Geometry check sheet. Reference: drawing and pictorial views, mm from the part's lowest x, y, z. A direction names the side the tool comes from. Round coordinates to 2 decimals unless told otherwise and drop trailing zeros. Order: outer loops, then holes, each group sorted by start corner. A loop starts at its lowest first (then second) coordinate and runs counter-clockwise, first axis right, second up. Notation, with made-up numbers: (-29.5, 54.5) -> (-4.5, 54.5) arc R25 ccw to (-4.5, 76.5) -> close; hole circle Ø7 at (44, 77.25). An arc over 180 degrees is marked (long way). Return JSON: item names as keys, results as strings. Group by question number.
1) Scan lines: L1, parallel to Z at x = 15, y = 1.5; L2, parallel to X at y = 0.8, z = 13; L3, parallel to X at y = 29.45, z = 20. Record each from-to range of solid material in increasing order.
2) Section check D-D on z = 17.5. Enter the section's corners in (x, y).
3) Depth check by flat-ended pin: pin 1 (2.5 mm diameter, centred on x = 25, z = 20, fed in from +Y). Enter the tip coordinate at first touch or a pass-through.
4) Section check A-A on y = 7.25. Enter the section's corners in (x, z).
5) Tool access check on the marked faces 1 and 2. Record the directions out of +Z, -Z, +X, -X, +Y, -Y that give a thin tool (end or side, any length) a straight path to the whole face; none if there is none.
6) Section check B-B on x = 5. Enter the section's corners in (y, z), plus the area to 3 significant figures.
7) Draft check along X on the marked faces 3, 4 and 5. Enter one of: pulls with the +X half, pulls with the -X half, needs draft (parallel to the pull), parting line crosses it, or undercut.
8) Section check C-C on z = 3.5. Enter the section's corners in (x, y), plus the area to 3 significant figures.
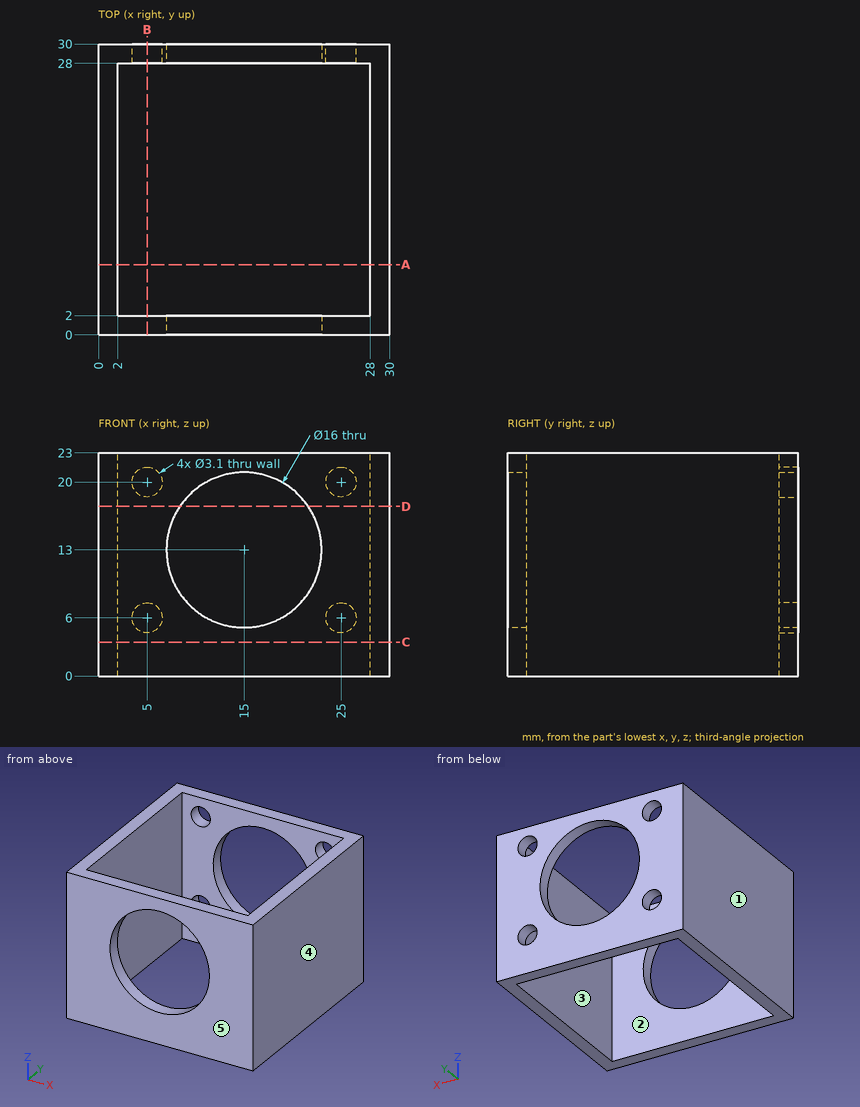
Check result:
{
 "1": {"L1": "0 to 5, 21 to 23", "L2": "0 to 7, 23 to 30", "L3": "0 to 3.45, 6.55 to 11.13, 18.87 to 23.45, 26.55 to 30"},
 "2": {"outline": "(0, 0) -> (8.39, 0) -> (8.39, 2) -> (2, 2) -> (2, 28) -> (8.39, 28) -> (8.39, 30) -> (0, 30) -> close; (21.61, 0) -> (30, 0) -> (30, 30) -> (21.61, 30) -> (21.61, 28) -> (28, 28) -> (28, 2) -> (21.61, 2) -> close"},
 "3": {"pin 1": "y = 2"},
 "4": {"outline": "(0, 0) -> (2, 0) -> (2, 23) -> (0, 23) -> close; (28, 0) -> (30, 0) -> (30, 23) -> (28, 23) -> close"},
 "5": {"face 1": "+Z, -Z, -X, +Y, -Y", "face 2": "+Z, -Z"},
 "6": {"outline": "(0, 0) -> (2, 0) -> (2, 23) -> (0, 23) -> close; (28, 0) -> (30, 0) -> (30, 4.45) -> (28, 4.45) -> close; (28, 7.55) -> (30, 7.55) -> (30, 18.45) -> (28, 18.45) -> close; (28, 21.55) -> (30, 21.55) -> (30, 23) -> (28, 23) -> close", "area": "79.6 mm^2"},
 "7": {"face 3": "undercut", "face 4": "pulls with the +X half", "face 5": "needs draft"},
 "8": {"outline": "(0, 0) -> (30, 0) -> (30, 30) -> (0, 30) -> close; hole (2, 2) -> (28, 2) -> (28, 28) -> (2, 28) -> close", "area": "224 mm^2"}
}
